Read the model definition and answer for the solid it produces. Units are mm, in the model's axes. A direction names the side the tool comes from. Coordinates: 2 decimals unless noted, no trailing zeros. Write each loop counter-clockwise with the first axis right and the second up, starting at its lowest first coordinate (ties: lowest second). Pieces come first, ordered by that corner, then holes. Notation, with made-up numbers: (65.5, 12) -> (94.5, 12) arc R18 cw to (94.5, 32) -> close; hole circle Ø6 at (-20.75, 4.25). An arc over 180 degrees is marked (long way). Return JSON: item names as keys, results as strings.
from build123d import *

# Parameters (mm, degrees)
F0_R     = 12.7
F1_DEPTH = 25.4
F2_R     = 31.75
F2_R_2   = 12.7
F3_DEPTH = 12.7
F5_DEPTH = 25.4


with BuildPart() as f1:
    # F0 (on Top) → F1 (new body)
    with BuildSketch(Plane.XY):
        Circle(F0_R)
        with BuildLine():
            ThreePointArc((1.7145, 6.114163), (0, -6.35), (-1.7145, 6.114163))
            Line((-1.7145, 6.114163), (-1.7145, 9.289163))
            Line((-1.7145, 9.289163), (1.7145, 9.289163))
            Line((1.7145, 9.289163), (1.7145, 6.114163))
        make_face(mode=Mode.SUBTRACT)
    extrude(amount=F1_DEPTH)

    # F2 (on face) → F3 (join)
    with BuildSketch(Plane(origin=(0, 0, 0), x_dir=(1, 0, 0), z_dir=(0, 0, -1))):
        Circle(F2_R)
        Circle(F2_R_2, mode=Mode.SUBTRACT)
    extrude(amount=-F3_DEPTH)

    # F4 (on face) → F5 (cut)
    with BuildSketch(Plane.XY.offset(12.7)):
        with BuildLine():
            ThreePointArc((-14.514286, 20.844556), (-15.305569, 16.424701), (-10.885714, 15.633417))
            ThreePointArc((-10.885714, 15.633417), (0, 19.05), (10.885714, 15.633417))
            ThreePointArc((10.885714, 15.633417), (15.305569, 16.424701), (14.514286, 20.844556))
            ThreePointArc((14.514286, 20.844556), (0, 25.4), (-14.514286, 20.844556))
        make_face()
        with BuildLine():
            ThreePointArc((-10.794772, -22.992018), (-6.571423, -21.467362), (-8.096079, -17.244014))
            ThreePointArc((-8.096079, -17.244014), (-16.497784, -9.525), (-18.981793, 1.610597))
            ThreePointArc((-18.981793, 1.610597), (-21.876993, 5.042662), (-25.309058, 2.147462))
            ThreePointArc((-25.309058, 2.147462), (-21.997045, -12.7), (-10.794772, -22.992018))
        make_face()
        with BuildLine():
            ThreePointArc((25.309058, 2.147462), (21.876993, 5.042662), (18.981793, 1.610597))
            ThreePointArc((18.981793, 1.610597), (16.497784, -9.525), (8.096079, -17.244014))
            ThreePointArc((8.096079, -17.244014), (6.571423, -21.467362), (10.794772, -22.992018))
            ThreePointArc((10.794772, -22.992018), (21.997045, -12.7), (25.309058, 2.147462))
        make_face()
    extrude(amount=-F5_DEPTH, mode=Mode.SUBTRACT)


solid = f1.part
1. Consider L1, parallel to Y at x = 0, z = 6.75; L2, parallel to Y at x = 0, z = 16.5; L3, parallel to X at y = -16.5, z = 11. Determine where each line is inside the solid, lowest interval first.
Taken from the geometry:
{"L1": "y = -31.75 to -6.35, 9.29 to 19.05, 25.4 to 31.75", "L2": "y = -12.7 to -6.35, 9.29 to 12.7", "L3": "x = -27.13 to -19.31, -9.52 to 9.52, 19.31 to 27.13"}
2. The part is cut by section B-B (x = 0). Determine the outline of the cut face in (y, z), then the cut area to 3 significant figures.
Taken from the geometry:
{"outline": "(-31.75, 0) -> (-6.35, 0) -> (-6.35, 25.4) -> (-12.7, 25.4) -> (-12.7, 12.7) -> (-31.75, 12.7) -> close; (9.29, 0) -> (19.05, 0) -> (19.05, 12.7) -> (12.7, 12.7) -> (12.7, 25.4) -> (9.29, 25.4) -> close; (25.4, 0) -> (31.75, 0) -> (31.75, 12.7) -> (25.4, 12.7) -> close", "area": "651 mm2"}
3. A tool of negligible diameter and unlimited length cuts with its end or side. For faces 5 (the face through (14, 0, 12.7)), 6 (the face through (1.714, 8, 13)), from which of +Z, -Z, +X, -X, +Y, -Y can it reach the whole face along a straight path? Write none if from no direction.
Taken from the geometry:
{"face 5": "+Z", "face 6": "+Z, -Z"}
4. The part is cut by section D-D (z = 4). Count the separate pieces of the cut face and the enclosed holes in it, then the cut area to 3 significant figures.
Taken from the geometry:
{"separate pieces": "1", "enclosed holes": "4", "area": "2,420 mm2"}
5. The part is cut by section C-C (z = 20.25). Determine the outline of the cut face in (x, y), then the cut area to 3 significant figures.
Taken from the geometry:
{"outline": "circle Ø25.4 at (0, 0); hole (-1.71, 6.11) arc R6.35 ccw (long way) to (1.71, 6.11) -> (1.71, 9.29) -> (-1.71, 9.29) -> close", "area": "370 mm2"}
6. For a pull along Y with two mould halves and no side action, classify faces 1 (the face through (-16.416, -9.665, 6.439)), 2 (the face through (7, 0, 0)), 3 (the face through (-6.883, 30.995, 6.261)), 4 (the face through (21.888, -12.887, 6.439)) as +Y half, -Y half, draft (parallel to the pull), parting line (faces both ways), or undercut.
Taken from the geometry:
{"face 1": "undercut", "face 2": "draft", "face 3": "parting line", "face 4": "undercut"}
7. The part is cut by section A-A (y = 0). Determine the outline of the cut face in (x, z), then the cut area to 3 significant figures.
Taken from the geometry:
{"outline": "(-31.75, 0) -> (-25.4, 0) -> (-25.4, 12.7) -> (-31.75, 12.7) -> close; (-19.05, 0) -> (-6.35, 0) -> (-6.35, 25.4) -> (-12.7, 25.4) -> (-12.7, 12.7) -> (-19.05, 12.7) -> close; (6.35, 0) -> (19.05, 0) -> (19.05, 12.7) -> (12.7, 12.7) -> (12.7, 25.4) -> (6.35, 25.4) -> close; (25.4, 0) -> (31.75, 0) -> (31.75, 12.7) -> (25.4, 12.7) -> close", "area": "645 mm2"}
8. Flat-ended cylindrical pins translate along their axes: pin 1 Ø6 at (y, z) = (-4, 17) entering from +X; pin 2 Ø8 at (x, z) = (-6.5, 7) entering from -Y; pin 3 Ø1 at (y, z) = (7, 7.5) entering from +X; pin 4 Ø16.5 at (x, y) = (0, 0) entering from -Z. Find the tip coordinate at first contact, or state that the pin passes through.
Taken from the geometry:
{"pin 1": "stops at x = 12.66", "pin 2": "stops at y = -31.65", "pin 3": "stops at x = 31.08", "pin 4": "stops at z = 0"}
